```python
from build123d import *

# Parameters (mm, degrees)
ESQUISSE1_W                                 = 100
ESQUISSE1_H                                 = 100
BOSS_EXTRU_1_DEPTH                          = 1.6
FRAISAGE_POUR_VIS_T_TE_FRAIS_E_M31_AT_COUNT = 2
FRAISAGE_POUR_VIS_T_TE_FRAIS_E_M31_AT_PITCH = 90
FRAISAGE_POUR_VIS_T_TE_FRAIS_E_M31_2_COUNT  = 2
FRAISAGE_POUR_VIS_T_TE_FRAIS_E_M31_2_PITCH  = 127.279220614
FRAISAGE_POUR_VIS_T_TE_FRAIS_E_M31_3_COUNT  = 2
FRAISAGE_POUR_VIS_T_TE_FRAIS_E_M31_3_PITCH  = 90
ESQUISSE4_R                                 = 1.5
ESQUISSE4_R_2                               = 5.05
ESQUISSE4_R_3                               = 1.95
ENL_V_MAT_EXTRU_1_DEPTH                     = 2.6


with BuildPart() as part:
    # Esquisse1 → Boss.-Extru.1 (new body)
    with BuildSketch(Plane.XY):
        with Locations((50, 50)):
            Rectangle(ESQUISSE1_W, ESQUISSE1_H)
    extrude(amount=BOSS_EXTRU_1_DEPTH)

    # Esquisse3 → Fraisage pour vis à tête fraisée M31 (revolve, cut)
    with BuildSketch(Plane(origin=(5, 95, 1.6), x_dir=(0, -1, 0), z_dir=(1, 0, 0))):
        Polygon((0, 0), (0, 1.6), (1.8, 1.6), (1.8, 1.35), (3.15, 0), align=None)
    fraisage_pour_vis_t_te_frais_e_m31 = revolve(axis=Axis((5, 95, 7.95), (0, 0, -1)), mode=Mode.SUBTRACT)

    # Fraisage pour vis à tête fraisée M31 at: Fraisage pour vis à tête fraisée M31 ×2
    with Locations(*[(i * FRAISAGE_POUR_VIS_T_TE_FRAIS_E_M31_AT_PITCH, 0, 0) for i in range(1, FRAISAGE_POUR_VIS_T_TE_FRAIS_E_M31_AT_COUNT)]):
        add(fraisage_pour_vis_t_te_frais_e_m31, mode=Mode.SUBTRACT)

    # Fraisage pour vis _ t_te frais_e M31 2: Fraisage pour vis à tête fraisée M31 ×2
    with Locations(*[Vector(0.707106781, -0.707106781, 0) * (i * FRAISAGE_POUR_VIS_T_TE_FRAIS_E_M31_2_PITCH) for i in range(1, FRAISAGE_POUR_VIS_T_TE_FRAIS_E_M31_2_COUNT)]):
        add(fraisage_pour_vis_t_te_frais_e_m31, mode=Mode.SUBTRACT)

    # Fraisage pour vis _ t_te frais_e M31 3: Fraisage pour vis à tête fraisée M31 ×2
    with Locations(*[(0, -i * FRAISAGE_POUR_VIS_T_TE_FRAIS_E_M31_3_PITCH, 0) for i in range(1, FRAISAGE_POUR_VIS_T_TE_FRAIS_E_M31_3_COUNT)]):
        add(fraisage_pour_vis_t_te_frais_e_m31, mode=Mode.SUBTRACT)

    # Esquisse4 → Enlèv. mat.-Extru.1 (cut, through all)
    with BuildSketch(Plane.XY.offset(1.6)):
        with Locations((11.557, 24.13)):
            Circle(ESQUISSE4_R)
        with Locations((11.557, 29.13)):
            Circle(ESQUISSE4_R)
        with Locations((15.887127019, 26.63)):
            Circle(ESQUISSE4_R)
        with Locations((15.887127019, 21.63)):
            Circle(ESQUISSE4_R)
        with Locations((11.557, 19.13)):
            Circle(ESQUISSE4_R)
        with Locations((7.226872981, 21.63)):
            Circle(ESQUISSE4_R)
        with Locations((7.226872981, 26.63)):
            Circle(ESQUISSE4_R)
        with Locations((12.5, 75)):
            Circle(ESQUISSE4_R_2)
        with Locations((12.5, 60)):
            Circle(ESQUISSE4_R_2)
        with Locations((12.5, 45)):
            Circle(ESQUISSE4_R_2)
        with Locations((25, 75)):
            Circle(ESQUISSE4_R_3)
        with Locations((24.07180174, 59.869246014)):
            Circle(ESQUISSE4_R_3)
        with Locations((24.07180174, 44.869246014)):
            Circle(ESQUISSE4_R_3)
    extrude(amount=-ENL_V_MAT_EXTRU_1_DEPTH, mode=Mode.SUBTRACT)


solid = part.part
```
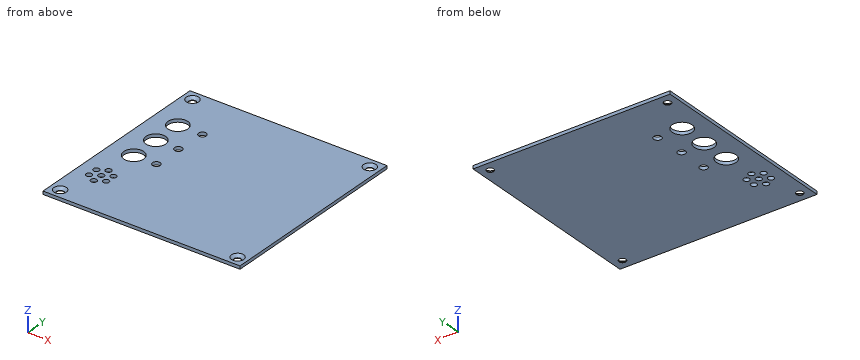
Could you check a few things on this model? Use its own coordinates, in mm. Round coordinates to 2 decimals unless told otherwise and drop trailing zeros. Loops run counter-clockwise (first coordinate to the right, second up) from the corner with the lowest first, then second, coordinate; pieces in that order, holes last. Notation, with made-up numbers: M -22,7 L 29,7 A23 cw 29,23 Z; hole C 4.5,7 d7. An arc over 180 degrees is marked long. Answer as CSV lines item,"result".
1) Imagine slicing it at A-A on y = 95. List the corners of the cut face in (x, z) for me, and give its area (3 significant figures).
From the geometry:
outline,"M 0,0 L 3.2,0 L 3.2,0.25 L 1.85,1.6 L 0,1.6 Z; M 6.8,0 L 93.2,0 L 93.2,0.25 L 91.85,1.6 L 8.15,1.6 L 6.8,0.25 Z; M 96.8,0 L 100,0 L 100,1.6 L 98.15,1.6 L 96.8,0.25 Z"
area,"145 mm^2"
2) If I drill on probe 1 along Y at (x, z) = (5, 0.2); probe 2 along X at (y, z) = (73, 0.3); probe 3 along X at (y, z) = (48, 1.45), over which ranges is the centre line in solid material (lowest first)?
From the geometry:
probe 1,"0 to 3.2, 6.8 to 93.2, 96.8 to 100"
probe 2,"0 to 7.86, 17.14 to 100"
probe 3,"0 to 8.44, 16.56 to 100"
